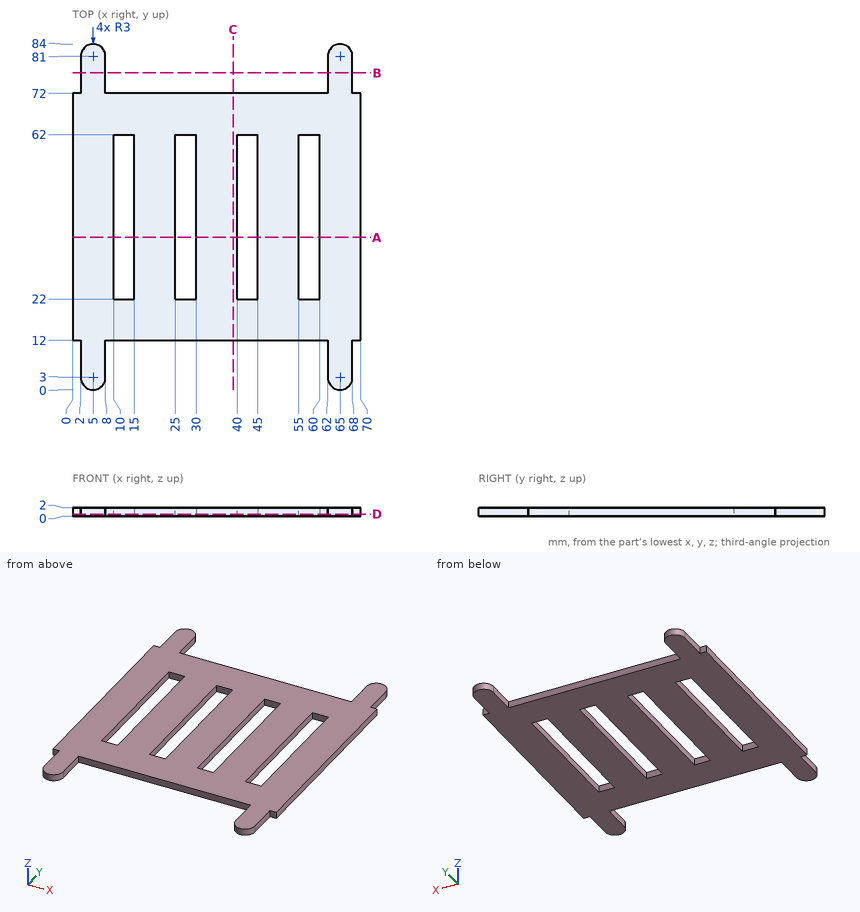
Verification items for this drawing (mm, ordinates from the low corner). Round coordinates to 2 decimals unless told otherwise and drop trailing zeros. Loops run counter-clockwise (first coordinate to the right, second up) from the corner with the lowest first, then second, coordinate; pieces in that order, holes last. Notation, with made-up numbers: (85.5, 51) -> (139.5, 51) arc R6 cw to (139.5, 62) -> close; hole circle Ø6 at (-18.5, -37.5). An arc over 180 degrees is marked (long way). Answer in a Markdown table with one row per item.
Q1. Go/stop test with flat-tipped pins: P1, Ø1, axis at y = 75.5, z = 1, coming from the +X side; P2, Ø0.6, axis at y = 75, z = 1, coming from the -X side; P3, Ø1, axis at x = 69, z = 1, coming from the +Y side. Record where each tip stops, or that it passes through.
Data:
| item | result |
|---|---|
| P1 | stops at x = 68 |
| P2 | stops at x = 2 |
| P3 | stops at y = 72 |
Q2. Sectioned sample at A-A on y = 37. Enter the section's corners in (x, z).
Data:
| item | result |
|---|---|
| outline | (0, 0) -> (10, 0) -> (10, 2) -> (0, 2) -> close; (15, 0) -> (25, 0) -> (25, 2) -> (15, 2) -> close; (30, 0) -> (40, 0) -> (40, 2) -> (30, 2) -> close; (45, 0) -> (55, 0) -> (55, 2) -> (45, 2) -> close; (60, 0) -> (70, 0) -> (70, 2) -> (60, 2) -> close |
Q3. Sectioned sample at D-D on z = 0.45. Give the number of separate pieces and of enclosed holes in the cut face, then the cut area to 3 significant figures.
Data:
| item | result |
|---|---|
| separate pieces | 1 |
| enclosed holes | 4 |
| area | 3,670 mm^2 |
Q4. Sectioned sample at B-B on y = 77. Enter the section's corners in (x, z), then the cut area to 3 significant figures.
Data:
| item | result |
|---|---|
| outline | (2, 0) -> (8, 0) -> (8, 2) -> (2, 2) -> close; (62, 0) -> (68, 0) -> (68, 2) -> (62, 2) -> close |
| area | 24.0 mm^2 |
Q5. Sectioned sample at C-C on x = 39. Enter the section's corners in (y, z).
Data:
| item | result |
|---|---|
| outline | (12, 0) -> (72, 0) -> (72, 2) -> (12, 2) -> close |
Q6. Thickness scan on L1, parallel to X at y = 61.5, z = 1.6; L2, parallel to Y at x = 57.5, z = 0.2; L3, parallel to X at y = 8, z = 1.8. Record the ranges inside material, lowest first.
Data:
| item | result |
|---|---|
| L1 | x = 0 to 10, 15 to 25, 30 to 40, 45 to 55, 60 to 70 |
| L2 | y = 12 to 22, 62 to 72 |
| L3 | x = 2 to 8, 62 to 68 |
